Here's how the part is built. I have some questions about the finished solid (model axes, mm). Face numbers are marked on the shaded views. A direction names the side the tool comes from. Round coordinates to 2 decimals unless told otherwise and drop trailing zeros. Loops run counter-clockwise (first coordinate to the right, second up) from the corner with the lowest first, then second, coordinate; pieces in that order, holes last. Notation, with made-up numbers: M 32,89.5 L 74,89.5 A16 ccw 74,100.5 Z; hole C 88.5,50.25 d6. An arc over 180 degrees is marked long. Put each result on its own line as item: value. Start each with the question number.
```python
from build123d import *

# Parameters (mm, degrees)
F1_DEPTH    = 38
F3_DEPTH    = 11
F5_DEPTH    = 11
F6_W        = 8
F6_H        = 48.4886
F7_DEPTH    = 48.4886
F8_T4_DEPTH = 265.1682987966


# Not quite as in the source:
# - a fillet or chamfer that OpenCascade refuses, or shapes differently, is made with other operations: its cross-section is extruded or revolved along the edge and cut away or added


with BuildPart() as f1:
    # F0 (on Front) → F1 (new body)
    with BuildSketch(Plane.XZ):
        Polygon((0, 49), (0, 0), (49, 0), (49, 11), (11, 11), (11, 49), align=None)
    extrude(amount=F1_DEPTH)

    # F2 (on face) → F3 (join)
    with BuildSketch(Plane(origin=(0, 0, 0), x_dir=(0, -1, 0), z_dir=(-1, 0, 0))):
        with BuildLine():
            Line((0, 49), (38, 49))
            ThreePointArc((38, 49), (19, 68), (0, 49))
        make_face()
    extrude(amount=-F3_DEPTH)

    # F4 (on face) → F5 (join)
    with BuildSketch(Plane.XY.offset(11)):
        with BuildLine():
            Line((49, 0), (49, -38))
            ThreePointArc((49, -38), (68, -19), (49, 0))
        make_face()
    extrude(amount=-F5_DEPTH)

    # F6 (on face) → F7 (join)
    with BuildSketch(Plane.YZ.offset(11)):
        with Locations((-19, 35.2443)):
            Rectangle(F6_W, F6_H)
    extrude(amount=F7_DEPTH)

    # F8: chamfer of 50 on 1 edges, made by hand


with BuildPart() as f8_tool2:
    # F8_s3 → F8_t4 (new body)
    with BuildSketch(Plane.XZ.offset(-113.5841493983)):
        Polygon((59.4886, 9.4886), (9.4886, 59.4886), (59.4886, 59.4886), align=None)
    extrude(amount=F8_T4_DEPTH)

    split(bisect_by=Plane.XY.offset(11), keep=Keep.TOP)

    split(bisect_by=Plane.YZ.offset(11), keep=Keep.TOP)


with BuildPart() as f1_1:
    add(f1.part)

    # F8_t1: cut F8_tool2
    add(f8_tool2.part, mode=Mode.SUBTRACT)


solid = f1_1.part
```
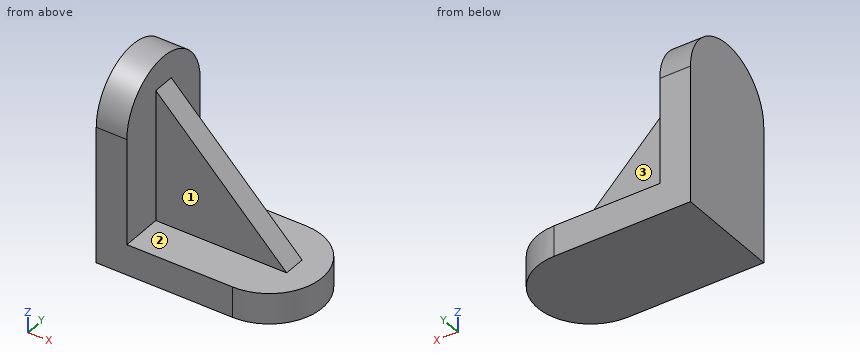
1) Suppose I cut it at B-B (x = 44.5). Write out the boundary of the cut face in (y, z), plus the area to 3 significant figures.
2) On a 3-axis mill with a long thin cutter (end or side, diameter ignored), from which of +Z, -Z, +X, -X, +Y, -Y can I reach the whole of each face in a straight line? I mean the marked faces 1, 2 and 3. Say none if no direction works.
3) If I drill on probe 1 along Z at (x, y) = (46, -3.5); probe 2 along Y at (x, z) = (30, 16), over which ranges is the centre line in solid material (lowest first)? Write a range as from..to.
4) Suppose I cut it at D-D (z = 6). Write out the boundary of the cut face in (x, y).
5) Suppose I cut it at A-A (y = -19). Write out the boundary of the cut face in (x, z).
6) I'm going to push flat-ended pins straight in: P1, Ø19, axis at x = 39.5, y = -21, coming from the +Z side; P2, Ø4, axis at x = 12.5, y = -31.5, coming from the +Z side; P3, Ø4, axis at x = 61, y = -14, coming from the -Z side; P4, Ø5, axis at x = 25.5, y = -11.5, coming from the +Z side. Where does each tip first touch, or does it pass through?
7) Suppose I cut it at C-C (z = 53). Write out the boundary of the cut face in (x, y), plus the area to 3 significant figures.
Results are:
1. outline: M -38,0 L 0,0 L 0,11 L -15,11 L -15,24.48 L -23,24.48 L -23,11 L -38,11 Z
1. area: 526 mm²
2. face 1: +Z, +X, -Y
2. face 2: +Z, +X
2. face 3: +Z, +X, +Y
3. probe 1: 0..11
3. probe 2: -23..-15
4. outline: M 0,-38 L 49,-38 A19 ccw 49,0 L 0,0 Z
5. outline: M 0,0 L 68,0 L 68,11 L 57.98,11 L 11,57.98 L 11,68 L 0,68 Z
6. P1: z = 38.98
6. P2: z = 64.36
6. P3: z = 0
6. P4: z = 11
7. outline: M 0,-37.57 L 11,-37.57 L 11,-23 L 15.98,-23 L 15.98,-15 L 11,-15 L 11,-0.43 L 0,-0.43 Z
7. area: 448 mm²
